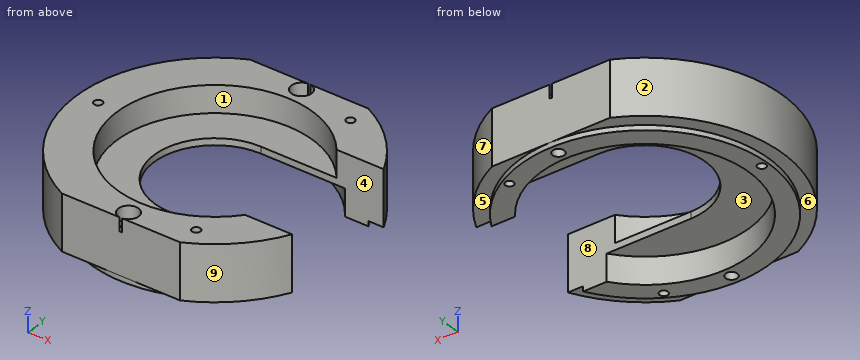
```python
from build123d import *

# Parameters (mm, degrees)
SKETCH_1_R                   = 41
EXTRUDE_1_DEPTH              = 16.5
SKETCH_2_R                   = 36.975
EXTRUDE_2_DEPTH              = 1.5
SKETCH_4_W                   = 50
SKETCH_4_H                   = 6.84002239
CUT_EXTRUDE_1_DEPTH          = 61.712436947
SKETCH_5_R                   = 31
CUT_EXTRUDE_3_DEPTH          = 8
SKETCH_6_R                   = 29
CUT_EXTRUDE_4_DEPTH          = 8
CUT_EXTRUDE_5_DEPTH          = 57.108382841
CUT_EXTRUDE_5_DEPTH_BACK     = 57.108382841
HOLE_WIZARD_M3_3_D           = 3.5
HOLE_WIZARD_M3_3_CBORE_D     = 6
HOLE_WIZARD_M3_3_CBORE_DEPTH = 4
HOLE_WIZARD_M3_1_D           = 2.5
PATTERN_CIRCULAR_1_COUNT     = 3


with BuildPart() as part:
    # 草图1 → 凸台-拉伸1 (new body)
    with BuildSketch(Plane.XY):
        Circle(SKETCH_1_R)
    extrude(amount=EXTRUDE_1_DEPTH)

    # 草图2 → 凸台-拉伸2 (add)
    with BuildSketch(Plane(origin=(0, 0, 0), x_dir=(-1, 0, 0), z_dir=(0, 0, -1))):
        Circle(SKETCH_2_R)
    extrude(amount=EXTRUDE_2_DEPTH)

    # 草图4 → 切除-拉伸1 (cut, through all)
    with BuildSketch(Plane(origin=(0, 0, -1.5), x_dir=(-1, 0, 0), z_dir=(0, 0, -1))):
        with Locations((0, 40.395011195)):
            Rectangle(SKETCH_4_W, SKETCH_4_H)
        with Locations((0, -40.395011195)):
            Rectangle(SKETCH_4_W, SKETCH_4_H)
    extrude(amount=-CUT_EXTRUDE_1_DEPTH, mode=Mode.SUBTRACT)

    # 草图5 → 切除-拉伸3 (cut)
    with BuildSketch(Plane(origin=(0, 0, -1.5), x_dir=(-1, 0, 0), z_dir=(0, 0, -1))):
        Circle(SKETCH_5_R)
    extrude(amount=-CUT_EXTRUDE_3_DEPTH, mode=Mode.SUBTRACT)

    # 草图6 → 切除-拉伸4 (cut)
    with BuildSketch(Plane.XY.offset(16.5)):
        Circle(SKETCH_6_R)
    extrude(amount=-CUT_EXTRUDE_4_DEPTH, mode=Mode.SUBTRACT)

    # 草图7 → 切除-拉伸5 (cut, two sides: drawn at the far end of the back side and taken through both)
    with BuildSketch(Plane.XY.offset(8.5).offset(-CUT_EXTRUDE_5_DEPTH_BACK)):
        with BuildLine():
            Line((0, 18), (36.837480913, 18))
            ThreePointArc((36.837480913, 18), (41, 0), (36.837480913, -18))
            Line((36.837480913, -18), (0, -18))
            ThreePointArc((0, -18), (-18, 0), (0, 18))
        make_face()
    extrude(amount=CUT_EXTRUDE_5_DEPTH + CUT_EXTRUDE_5_DEPTH_BACK, mode=Mode.SUBTRACT)

    # M3 六角头螺栓的柱形沉头孔3 (through all)
    with Locations(Plane(origin=(0, 34, 16.5), x_dir=(1, 0, 0), z_dir=(0, 0, 1))):
        with Locations((0, 0), (0, -68)):
            CounterBoreHole(HOLE_WIZARD_M3_3_D / 2, HOLE_WIZARD_M3_3_CBORE_D / 2, HOLE_WIZARD_M3_3_CBORE_DEPTH)

    # M3 螺纹孔1 (through all)
    with Locations(Plane(origin=(-35, 0, 16.5), x_dir=(1, 0, 0), z_dir=(0, 0, 1))):
        with Locations((0, 0)):
            hole_wizard_m3_1 = Hole(HOLE_WIZARD_M3_1_D / 2)

    # 阵列(圆周)1: M3 螺纹孔1 ×3 about axis
    pattern_circular_1_axis = Axis((0, 0, 0), (0, 0, 1))
    for i in range(1, PATTERN_CIRCULAR_1_COUNT):
        add(hole_wizard_m3_1.rotate(pattern_circular_1_axis, i * 360 / PATTERN_CIRCULAR_1_COUNT), mode=Mode.SUBTRACT)


solid = part.part
```
Can you work these out from the model? Positions are in its coordinate system, mm. Face numbers are marked on the shaded views. A direction names the side the tool comes from. Round coordinates to 2 decimals unless told otherwise and drop trailing zeros. Loops run counter-clockwise (first coordinate to the right, second up) from the corner with the lowest first, then second, coordinate; pieces in that order, holes last. Notation, with made-up numbers: M -10,-39.5 L 37,-39.5 A8 ccw 37,-26.5 Z; hole C 10.25,81 d5. An arc over 180 degrees is marked long. Write item = value, one per line. Start each with the question number.
(1) I need wall thicknesses on line 1 along Y through (x, z) = (0, 0.75) (3 decimals); line 2 along Y through (x, z) = (0, 13); line 3 along Y through (x, z) = (17, 7.5) (3 decimals). Which ranges of each line are inside material? Lowest first, please.
(2) Suppose I cut it at D-D on z = 15.5. Give the number of separate pieces and of enclosed holes in the cut face, plus the area to 3 significant figures.
(3) Suppose I cut it at B-B on x = -11. Write out the boundary of the cut face in (y, z) (3 decimals).
(4) Which directions (+Z, -Z, +X, -X, +Y, -Y) give clear straight access to the entire face, cutting with the end or side of a thin tool? Please do the marked faces 1, 2, 3, 4 and 5.
(5) I'm going to push flat-ended pins straight in: P1, Ø1.5, axis at x = -16.5, y = 0, coming from the -Z side; P2, Ø5, axis at y = -7, z = 5.5, coming from the -X side; P3, Ø8, axis at y = 4.5, z = 10, coming from the +X side; P4, Ø5, axis at x = 13, y = -21, coming from the -Z side. Where does each tip first touch, or does it pass through?
(6) Suppose I cut it at C-C on z = 9.75. Write out the boundary of the cut face in (x, y) (3 decimals), plus the area to 3 significant figures.
(7) Suppose I cut it at A-A on y = 0. Write out the boundary of the cut face in (x, z) (3 decimals), plus the area to 3 significant figures.
(8) If we mould it in two halves opening along Y, with no side actions, what happens to the marked faces 6, 7, 8 and 9? For each: released by +Y, released by -Y, zero draft, split by the parting line, or undercut.
Answer block:
q1.line_1 = -36.975 to -35.75, -32.25 to -31, 31 to 32.25, 35.75 to 36.975
q1.line_2 = -31 to -29, 29 to 31
q1.line_3 = -36.975 to -31.457, -29.165 to -18, 18 to 29.165, 31.457 to 36.975
q2.separate_pieces = 1
q2.enclosed_holes = 3
q2.area = 1,920 mm²
q3.outline = M -36.975,0 L -35.301,0 L -35.301,-1.5 L -28.983,-1.5 L -28.983,6.5 L -14.248,6.5 L -14.248,8.5 L -26.833,8.5 L -26.833,16.5 L -36.975,16.5 Z; M 14.248,6.5 L 28.983,6.5 L 28.983,-1.5 L 35.301,-1.5 L 35.301,0 L 36.975,0 L 36.975,16.5 L 26.833,16.5 L 26.833,8.5 L 14.248,8.5 Z
q4.face_1 = +Z
q4.face_2 = +Z, -Z, -X
q4.face_3 = -Z
q4.face_4 = +Z, -Z, +X
q4.face_5 = -Z, +X, +Y
q5.P1 = through
q5.P2 = -40.75
q5.P3 = -16.02
q5.P4 = 6.5
q6.outline = M -17.716,-36.975 L 17.716,-36.975 A41 ccw 36.837,-18 L 22.738,-18 A29 cw long 22.738,18 L 36.837,18 A41 ccw 17.716,36.975 L -17.716,36.975 A41 ccw Z; hole C -35,0 d2.5; hole C 0,-34 d3.5; hole C 0,34 d3.5; hole C 17.5,-30.311 d2.5; hole C 17.5,30.311 d2.5
q6.area = 1,960 mm²
q7.outline = M -41,0 L -36.975,0 L -36.975,-1.5 L -36.25,-1.5 L -36.25,16.5 L -41,16.5 Z; M -33.75,-1.5 L -31,-1.5 L -31,6.5 L -18,6.5 L -18,8.5 L -29,8.5 L -29,16.5 L -33.75,16.5 Z
q7.area = 171 mm²
q8.face_6 = zero draft
q8.face_7 = released by +Y
q8.face_8 = undercut
q8.face_9 = released by -Y
